The model under review builds one solid part; all positions refer to its coordinate system, in mm. A direction names the side the tool comes from. Round coordinates to 2 decimals unless told otherwise and drop trailing zeros. Order: outer loops, then holes, each group sorted by start corner. A loop starts at its lowest first (then second) coordinate and runs counter-clockwise, first axis right, second up. Notation, with made-up numbers: (15, 60.25) -> (37, 60.25) arc R16 cw to (37, 80.25) -> close; hole circle Ø5 at (66, -28.75). An arc over 180 degrees is marked (long way). Use a Markdown table: item, result. Add a question column.
```python
from build123d import *

# Parameters (mm, degrees)
SKETCH_1_R      = 1
EXTRUDE_1_DEPTH = 1.5
SKETCH_2_W      = 7.5
SKETCH_2_H      = 6
EXTRUDE_2_DEPTH = 2.5


with BuildPart() as part:
    # Эскиз1 → Бобышка-Вытянуть1 (new body)
    with BuildSketch(Plane.XY):
        Polygon((16.5, 12), (-16.5, 12), (-16.5, -12), (1, -12), (1, -10.5), (12.5, -10.5), (12.5, -12), (16.5, -12), align=None)
        with Locations((-14.5, -10)):
            Circle(SKETCH_1_R, mode=Mode.SUBTRACT)
        with Locations((-7, -10)):
            Circle(SKETCH_1_R, mode=Mode.SUBTRACT)
        with Locations((-1, -10)):
            Circle(SKETCH_1_R, mode=Mode.SUBTRACT)
        with Locations((14.5, -10)):
            Circle(SKETCH_1_R, mode=Mode.SUBTRACT)
        with Locations((2.5, 10)):
            Circle(SKETCH_1_R, mode=Mode.SUBTRACT)
        with Locations((11.5, 10)):
            Circle(SKETCH_1_R, mode=Mode.SUBTRACT)
    extrude(amount=-EXTRUDE_1_DEPTH)

    # Эскиз2 → Бобышка-Вытянуть2 (add)
    with BuildSketch(Plane.XY):
        with Locations((6.75, -8.5)):
            Rectangle(SKETCH_2_W, SKETCH_2_H)
    extrude(amount=EXTRUDE_2_DEPTH)


solid = part.part
```
Q1. For faces 1 (the face through (7, -10.5, -1)), 2 (the face through (3, -9, 1)), 3 (the face through (12.5, -11, -1)), 4 (the face through (10.5, -9, 1)), list the 3-axis set-ups (+Z, -Z, +X, -X, +Y, -Y) from which the entire face can be reached by the end or side of a thin tool; tool diameter is ignored.
Q2. Draft analysis for pull direction Y (two halves, no side actions). For faces 5 (the face through (7, -5.5, 1)), 6 (the face through (7, -8, 2.5)), 7 (the face through (15.454, -9.7, -0.74)), 8 (the face through (-7, -9, -1)), state which applies: released by +Y, released by -Y, zero draft, split by the parting line, or undercut.
Q3. Add section D-D, the plane y = 10. Give the boundary of the cut face in (x, z).
Q4. Add section B-B, the plane y = -10. Give the boundary of the cut face in (x, z).
Q5. Add section C-C, the plane z = -0.35. Give the boundary of the cut face in (x, y), then the cut area to 3 significant figures.
Q6. For pin 1 (0.8 mm diameter, centred on y = -10, z = 1.5, fed in from -X); pin 2 (0.8 mm diameter, centred on x = 6, y = -11, fed in from -Z); pin 3 (0.8 mm diameter, centred on x = 7, z = 1.5, fed in from -Y), all flat-tipped, find the tip position at first contact; note any pin that passes through.
Q7. To check wall thickness, follow line 1 along Y through (x, z) = (14.5, -1); line 2 along Z through (x, y) = (-6, 8.75). State the ranges of each line that lie inside material, in increasing order.
Q8. Add section A-A, the plane x = 11.5. Give the boundary of the cut face in (y, z), then the cut area to 4 significant figures.
Return value:
| question | item | result |
|---|---|---|
| 1 | face 1 | -Z, -Y |
| 1 | face 2 | +Z, -X, +Y, -Y |
| 1 | face 3 | +Z, -Z, -Y |
| 1 | face 4 | +Z, +X, +Y, -Y |
| 2 | face 5 | released by +Y |
| 2 | face 6 | zero draft |
| 2 | face 7 | undercut |
| 2 | face 8 | undercut |
| 3 | outline | (-16.5, -1.5) -> (1.5, -1.5) -> (1.5, 0) -> (-16.5, 0) -> close; (3.5, -1.5) -> (10.5, -1.5) -> (10.5, 0) -> (3.5, 0) -> close; (12.5, -1.5) -> (16.5, -1.5) -> (16.5, 0) -> (12.5, 0) -> close |
| 4 | outline | (-16.5, -1.5) -> (-15.5, -1.5) -> (-15.5, 0) -> (-16.5, 0) -> close; (-13.5, -1.5) -> (-8, -1.5) -> (-8, 0) -> (-13.5, 0) -> close; (-6, -1.5) -> (-2, -1.5) -> (-2, 0) -> (-6, 0) -> close; (0, -1.5) -> (13.5, -1.5) -> (13.5, 0) -> (10.5, 0) -> (10.5, 2.5) -> (3, 2.5) -> (3, 0) -> (0, 0) -> close; (15.5, -1.5) -> (16.5, -1.5) -> (16.5, 0) -> (15.5, 0) -> close |
| 5 | outline | (-16.5, -12) -> (1, -12) -> (1, -10.5) -> (12.5, -10.5) -> (12.5, -12) -> (16.5, -12) -> (16.5, 12) -> (-16.5, 12) -> close; hole circle Ø2 at (-14.5, -10); hole circle Ø2 at (-7, -10); hole circle Ø2 at (-1, -10); hole circle Ø2 at (2.5, 10); hole circle Ø2 at (11.5, 10); hole circle Ø2 at (14.5, -10) |
| 5 | area | 756 mm² |
| 6 | pin 1 | x = 3 |
| 6 | pin 2 | z = 0 |
| 6 | pin 3 | y = -11.5 |
| 7 | line 1 | -12 to -11, -9 to 12 |
| 7 | line 2 | -1.5 to 0 |
| 8 | outline | (-10.5, -1.5) -> (9, -1.5) -> (9, 0) -> (-10.5, 0) -> close; (11, -1.5) -> (12, -1.5) -> (12, 0) -> (11, 0) -> close |
| 8 | area | 30.75 mm² |
